For this review, take the finished solid that the model builds, in its own axes (mm). A direction names the side the tool comes from. Give positions to 0.01 mm unless a question says otherwise; leave off trailing zeros. Write each loop counter-clockwise with the first axis right and the second up, starting at its lowest first coordinate (ties: lowest second). Pieces come first, ordered by that corner, then holes. Notation, with made-up numbers: (17.25, 49) -> (40.25, 49) arc R11 ccw to (40.25, 60) -> close; hole circle Ø11 at (-34, -19.75). An arc over 180 degrees is marked (long way). Return JSON: item names as keys, results as strings.
from build123d import *

# Parameters (mm, degrees)
F1_DEPTH      = 2.286
F4_DEPTH      = 2.287
F5_DEPTH      = 6.35
F5_DEPTH_BACK = 2.286


# Not quite as in the source:
# - a feature names something its author has since deleted; it is built from what else it names


with BuildPart() as f1:
    # F0 (on Top) → F1 (new body)
    with BuildSketch(Plane.XY):
        Polygon((-39.7502322496, -19.8751161248), (-31.0001806734, -29.1251689516), (73.3058652154, -29.1251689516), (101.3186621261, 20.063493978), (101.3186621261, 25.3395497125), (78.8771229202, 34.0285638846), (72.3271246897, 39.6729167182), (52.3297434038, 47.023841916), (50.4247434038, 47.023841916), (21.8864718038, 47.023841916), (19.9814718038, 47.023841916), (-8.5567997962, 47.023841916), (-12.4402794499, 23.3751358177), (-17.5001015898, 6.8750406358), (-33.2501941145, 0), (-48.0002794499, -4.3750257881), align=None)
    extrude(amount=F1_DEPTH)

    # F3 (on face) → F4 (cut, through all)
    with BuildSketch(Plane.XY.offset(2.286)):
        Polygon((-1.4134727199, 27.9240615151), (-10.8518015695, 19.606512621), (-13.772583649, 9.942060765), (-8.389721466, -3.9236969292), (39.1813585612, 5.4958437045), align=None)
        Polygon((39.1813585612, 42.3302979083), (14.9339871262, 42.3302979083), (0.6105190133, 29.707708861), (39.1813585612, 8.3977252198), align=None)
        Polygon((59.9464575784, 35.9643820735), (41.7213585612, 42.3302979083), (41.7213585612, -3.8873157464), (74.8655756118, 26.1523920247), align=None)
        Polygon((94.1682944652, 13.4573999427), (77.0573760218, 24.7108910081), (62.4269453342, 11.4508444138), (82.0611413863, -7.8019792523), align=None)
        Polygon((97.8877921519, 22.7117055132), (69.8045753566, 32.5210017107), (95.4278561797, 15.6691089989), align=None)
        Polygon((60.5416469817, 9.7421357277), (41.7213585612, -7.3153184719), (41.7213585612, -25.5348474687), (71.9623257974, -25.5348474687), (80.7611698183, -10.0846454022), align=None)
        Polygon((39.1813585612, -25.5348474687), (39.1813585612, 2.906528429), (15.8625438549, -1.7108256973), align=None)
        Polygon((12.8853386979, -2.3003415321), (-7.4562708514, -6.3281798236), (0, -25.5348474687), (35.6271387151, -25.5348474687), align=None)
        Polygon((-2.7246861202, -25.5348474687), (-13.8299450744, 3.0712777777), (-29.3522901989, -25.5348474687), align=None)
        Polygon((-31.0001806734, -23.2460485454), (-17.5001015898, 1.6332432115), (-31.0001806734, -3.6563351177), (-41.1958687779, -9.0849860736), align=None)
        Polygon((11.0922382598, 42.3302979083), (-6.8430267274, 42.3302979083), (-8.8859712705, 26.1111650616), (-9.4571967621, 24.2210612772), align=None)
    extrude(amount=-F4_DEPTH, mode=Mode.SUBTRACT)

    # F2 (on face) → F5 (join, two sides)
    with BuildSketch(Plane.XY.offset(2.286)) as f5_sk:
        Polygon((75.6003040089, -19.9636537803), (71.829370857, -26.5851689516), (11.132148453, 7.9817182735), (33.3665214857, 47.023841916), (30.4435046989, 47.023841916), (10.9098193266, 12.7239514546), (10.9098193266, 23.5798310484), (-12.3775088144, 23.5798310484), (-12.4402794499, 23.3751358177), (-13.1564102749, 21.0398310484), (8.3698193266, 21.0398310484), (8.3698193266, -26.5851689516), (-28.1426806734, -26.5851689516), (-28.1426806734, 2.2294702333), (-30.6826806734, 1.1207400345), (-30.6826806734, -29.1251689516), (-28.1426806734, -29.1251689516), (8.3698193266, -29.1251689516), (10.9098193266, -29.1251689516), (10.9098193266, 5.1853172614), (71.1568181061, -29.1251689516), (73.3058652154, -29.1251689516), (77.8074757327, -21.2206314976), align=None)
        Polygon((91.6267699042, 8.177785698), (83.1421703125, -6.7206234376), (85.3493420363, -7.9776011549), (93.8339416279, 6.9208079807), align=None)
        Polygon((99.4828806371, 21.9726089716), (97.9116584905, 19.2136443169), (100.1188302143, 17.9566665996), (101.3186621261, 20.063493978), (101.3186621261, 25.3395497125), (78.8771229202, 34.0285638846), (72.3271246897, 39.6729167182), (61.2565125507, 43.7424116468), align=None)
    extrude(amount=F5_DEPTH)
    extrude(f5_sk.sketch, amount=-F5_DEPTH_BACK)


solid = f1.part
1. The part is to be moulded in two halves that separate along Y. For faces 4 (the flat face through (-40.522, -2.157, 1.127)), 5 (the flat face through (88, 0, 8.636)), 6 (the flat face through (-36.027, -6.333, 1.159)), say which applies: +Y half, -Y half, draft (parallel to the pull), parting line (faces both ways), or undercut.
Results found:
{"face 4": "+Y half", "face 5": "draft", "face 6": "undercut"}
2. Add section A-A, the plane z = 4. Count the separate pieces of the cut face and the enclosed holes in it, plus the area to 3 significant figures.
Results found:
{"separate pieces": "3", "enclosed holes": "0", "area": "793 mm²"}
3. Add section B-B, the plane x = 47.5. State the section outline as (y, z) points.
Results found:
{"outline": "(-29.13, 0) -> (-25.53, 0) -> (-25.53, 2.29) -> (-29.13, 2.29) -> close; (-15.65, 0) -> (-12.73, 0) -> (-12.73, 8.64) -> (-15.65, 8.64) -> close; (-2.08, 0) -> (1.35, 0) -> (1.35, 2.29) -> (-2.08, 2.29) -> close; (40.31, 0) -> (47.02, 0) -> (47.02, 2.29) -> (40.31, 2.29) -> close"}
4. To check wall thickness, follow probe 1 along Y at (x, z) = (-6, 6); probe 2 along X at (y, z) = (-6, 5.5); probe 3 along X at (y, z) = (-5, 5.25). State the ranges of each line that lie inside material, in increasing order.
Results found:
{"probe 1": "y = -29.13 to -26.59, 21.04 to 23.58", "probe 2": "x = -30.68 to -28.14, 8.37 to 10.91, 30.55 to 35.68, 83.55 to 86.48", "probe 3": "x = -30.68 to -28.14, 8.37 to 10.91, 28.79 to 33.93, 84.12 to 87.05"}
5. For pin 1 (1.5 mm diameter, centred on y = 0.5, z = 5.5, fed in from +X); pin 2 (4.5 mm diameter, centred on y = -10.5, z = 6, fed in from +X); pin 3 (0.7 mm diameter, centred on y = 18, z = 0.5, fed in from -X), all flat-tipped, find the tip position at first contact; note any pin that passes through.
Results found:
{"pin 1": "stops at x = 90.6", "pin 2": "stops at x = 47.54", "pin 3": "stops at x = -14.2"}
6. For faces 1 (the flat face through (40.61, -11.73, 4.38)), 2 (the flat face through (-8.2, -11.43, 1.16)), 3 (the flat face through (-10.47, 35.37, 1.13)), list the 3-axis set-ups (+Z, -Z, +X, -X, +Y, -Y) from which the entire face can be reached by the end or side of a thin tool; tool diameter is ignored.
Results found:
{"face 1": "+Z", "face 2": "+Z, -Z", "face 3": "+Z, -Z, -X, +Y"}
